```python
from build123d import *

# Parameters (mm, degrees)
PAD_DEPTH    = 12
SKETCH001_R  = 12
POCKET_DEPTH = 20


with BuildPart() as part:
    # Sketch → Pad (new body)
    with BuildSketch(Plane.YZ):
        Polygon((0, 0), (0, 110), (495, 110), (495, 0), (247.5, 0), align=None)
    extrude(amount=-PAD_DEPTH)

    # Sketch001 (on Face7 of Pad) → Pocket (cut)
    with BuildSketch(Plane(origin=(-12, 0, 0), x_dir=(0, -1, 0), z_dir=(-1, 0, 0))):
        with Locations((-197.5, 82)):
            Circle(SKETCH001_R)
        with Locations((-297.5, 82)):
            Circle(SKETCH001_R)
        with Locations((-347.5, 82)):
            Circle(SKETCH001_R)
        with Locations((-147.5, 82)):
            Circle(SKETCH001_R)
    extrude(amount=-POCKET_DEPTH, mode=Mode.SUBTRACT)


solid = part.part
```
The model under review builds one solid part; all positions refer to its coordinate system, in mm. Round coordinates to 2 decimals unless told otherwise and drop trailing zeros. Order: outer loops, then holes, each group sorted by start corner. A loop starts at its lowest first (then second) coordinate and runs counter-clockwise, first axis right, second up. Notation, with made-up numbers: (1.5, 82) - (30.5, 82) arc R6 cw to (30.5, 86) - close; hole circle Ø4 at (33.25, -7). An arc over 180 degrees is marked (long way). Answer in a Markdown table with one row per item.
(1) Take a section at C-C on x = -8.75. Write out the cut boundary in (y, z).
Result set:
| item | result |
|---|---|
| outline | (0, 0) - (495, 0) - (495, 110) - (0, 110) - close; hole circle Ø24 at (147.5, 82); hole circle Ø24 at (197.5, 82); hole circle Ø24 at (297.5, 82); hole circle Ø24 at (347.5, 82) |
(2) Take a section at A-A on z = 82. Write out the cut boundary in (x, y).
Result set:
| item | result |
|---|---|
| outline | (-12, 0) - (0, 0) - (0, 135.5) - (-12, 135.5) - close; (-12, 159.5) - (0, 159.5) - (0, 185.5) - (-12, 185.5) - close; (-12, 209.5) - (0, 209.5) - (0, 285.5) - (-12, 285.5) - close; (-12, 309.5) - (0, 309.5) - (0, 335.5) - (-12, 335.5) - close; (-12, 359.5) - (0, 359.5) - (0, 495) - (-12, 495) - close |
(3) Take a section at B-B on y = 297.5. Write out the cut boundary in (x, z).
Result set:
| item | result |
|---|---|
| outline | (-12, 0) - (0, 0) - (0, 70) - (-12, 70) - close; (-12, 94) - (0, 94) - (0, 110) - (-12, 110) - close |
(4) For line 1 (Z direction, x = -2.75, y = 347.5); line 2 (Y direction, x = -7.25, z = 91); line 3 (Y direction, x = -10, z = 78.5), list the stretches that pass through material, from the lowest coordinate up. Write a range as from..to.
Result set:
| item | result |
|---|---|
| line 1 | z = 0..70, 94..110 |
| line 2 | y = 0..139.56, 155.44..189.56, 205.44..289.56, 305.44..339.56, 355.44..495 |
| line 3 | y = 0..136.02, 158.98..186.02, 208.98..286.02, 308.98..336.02, 358.98..495 |
(5) Take a section at D-D on y = 348.5. Write out the cut boundary in (x, z), plus the area to 3 significant figures.
Result set:
| item | result |
|---|---|
| outline | (-12, 0) - (0, 0) - (0, 70.04) - (-12, 70.04) - close; (-12, 93.96) - (0, 93.96) - (0, 110) - (-12, 110) - close |
| area | 1,030 mm2 |
(6) Mouldability with a two-part tool opening along Z and no side actions: class faces 1 (the face through (-6.084, 307.023, 74.698)), 2 (the face through (-6, 244, 110)), 3 (the face through (-12, 251, 56)) as released by +Z, released by -Z, zero draft, split by the parting line, or undercut.
Result set:
| item | result |
|---|---|
| face 1 | undercut |
| face 2 | released by +Z |
| face 3 | zero draft |
